```python
from build123d import *

# Parameters (mm, degrees)
SKETCH1_W           = 46.3
SKETCH1_H           = 6.5
BOSS_EXTRUDE1_DEPTH = 59
FILLET1_R           = 1.25
SKETCH2_W           = 1.8
SKETCH2_H           = 3.75
CUT_EXTRUDE1_DEPTH  = 1.25
SKETCH3_W           = 1.7
SKETCH3_H           = 4.6
CUT_EXTRUDE2_DEPTH  = 0.4
FILLET2_R           = 0.25


with BuildPart() as part:
    # Sketch1 → Boss-Extrude1 (new body)
    with BuildSketch(Plane(origin=(0, 0, 0), x_dir=(1, 0, 0), z_dir=(0, 1, 0))):
        Rectangle(SKETCH1_W, SKETCH1_H)
    extrude(amount=BOSS_EXTRUDE1_DEPTH)

    # Fillet1
    fillet1_edges = [part.edges().sort_by_distance(p)[0] for p in [
        (23.15, 29.5, 3.25),
        (-23.15, 29.5, 3.25),
        (-23.15, 29.5, -3.25),
        (23.15, 29.5, -3.25),
    ]]
    fillet(fillet1_edges, radius=FILLET1_R)

    # Sketch2 → Cut-Extrude1 (cut)
    with BuildSketch(Plane(origin=(0, 59, 0), x_dir=(1, 0, 0), z_dir=(0, 1, 0))):
        with Locations((22.25, 0)):
            Rectangle(SKETCH2_W, SKETCH2_H)
        with BuildLine():
            Line((-21.85, 3.25), (-21.85, 1.875))
            Line((-21.85, 1.875), (-20.35, 1.875))
            Line((-20.35, 1.875), (-20.35, 0))
            Line((-20.35, 0), (-20.35, -1.875))
            Line((-20.35, -1.875), (-21.85, -1.875))
            Line((-21.85, -1.875), (-21.85, -3.25))
            Line((-21.85, -3.25), (-21.9, -3.25))
            ThreePointArc((-21.9, -3.25), (-22.783883476, -2.883883476), (-23.15, -2))
            Line((-23.15, -2), (-23.15, 2))
            ThreePointArc((-23.15, 2), (-22.783883476, 2.883883476), (-21.9, 3.25))
            Line((-21.9, 3.25), (-21.85, 3.25))
        make_face()
    extrude(amount=-CUT_EXTRUDE1_DEPTH, mode=Mode.SUBTRACT)

    # Sketch3 → Cut-Extrude2 (cut)
    with BuildSketch(Plane(origin=(0, 59, 0), x_dir=(1, 0, 0), z_dir=(0, 1, 0))):
        with Locations((-15.05, 0)):
            Rectangle(SKETCH3_W, SKETCH3_H)
        with Locations((-12.566666667, 0)):
            Rectangle(SKETCH3_W, SKETCH3_H)
        with Locations((-10.083333333, 0)):
            Rectangle(SKETCH3_W, SKETCH3_H)
        with Locations((-7.6, 0)):
            Rectangle(SKETCH3_W, SKETCH3_H)
    extrude(amount=-CUT_EXTRUDE2_DEPTH, mode=Mode.SUBTRACT)

    # Fillet2
    fillet2_edges = [part.edges().sort_by_distance(p)[0] for p in [
        (-13.416666667, 58.8, -2.3),
        (-11.716666667, 58.8, -2.3),
        (-11.716666667, 58.8, 2.3),
        (-13.416666667, 58.8, 2.3),
        (-10.933333333, 58.8, -2.3),
        (-9.233333333, 58.8, -2.3),
        (-9.233333333, 58.8, 2.3),
        (-10.933333333, 58.8, 2.3),
        (-8.45, 58.8, -2.3),
        (-6.75, 58.8, -2.3),
        (-6.75, 58.8, 2.3),
        (-8.45, 58.8, 2.3),
        (-14.2, 58.8, -2.3),
        (-14.2, 58.8, 2.3),
        (-15.9, 58.8, 2.3),
        (-15.9, 58.8, -2.3),
    ]]
    fillet(fillet2_edges, radius=FILLET2_R)


solid = part.part
```
CAD build for the part. Positions are in the model's coordinates, mm. A direction names the side the tool comes from. Round coordinates to 2 decimals unless told otherwise and drop trailing zeros. One line per question, with ' | ' between items.
Q1. Two-plate mould, pull along X, no slides. Class faces 6 (the flat face through (-23.15, 28, 0)), 7 (the flat face through (-15, 58.6, 0)), 8 (the flat face through (-22, 57.75, 0)): released by +X, released by -X, zero draft, split by the parting line, or undercut.
Completed:
face 6: released by -X | face 7: undercut | face 8: zero draft
Q2. Drop a flat-ended pin along its axis: pin 1 (1.4 mm diameter, centred on x = -10, z = 0, fed in from +Y). Give the stop position or say it passes through.
Completed:
pin 1: stops at y = 58.6
Q3. Probe probe 1 along X at (y, z) = (11, 2.75); probe 2 along X at (y, z) = (14.5, -2.5). List the from-to ranges inside material, lowest first.
Completed:
probe 1: x = -22.9 to 22.9 | probe 2: x = -23.05 to 23.05
Q4. Which spindle directions (+Z, -Z, +X, -X, +Y, -Y) get a long thin tool onto all of the face, cutting with end or side? Do faces 1 (the flat face through (22, 58, 1.875)), 2 (the flat face through (-21.85, 58, -3)), 3 (the flat face through (-21, 58, 1.875)), 4 (the flat face through (0, 29, 3.25)), 5 (the flat face through (-13, 58.6, 0)). Say none if no direction does.
Completed:
face 1: +X, +Y | face 2: +Z, -Z, -X, +Y | face 3: -X, +Y | face 4: +Z, +X, -X, +Y, -Y | face 5: +Y
